Verification items for the finished model (mm, model axes). Face numbers are marked on the shaded views. A direction names the side the tool comes from. Round coordinates to 2 decimals unless told otherwise and drop trailing zeros. Order: outer loops, then holes, each group sorted by start corner. A loop starts at its lowest first (then second) coordinate and runs counter-clockwise, first axis right, second up. Notation, with made-up numbers: (30, 82.25) -> (65, 82.25) arc R6 ccw to (65, 90.25) -> close; hole circle Ø2 at (-39, 45). An arc over 180 degrees is marked (long way). Return JSON: item names as keys, results as strings. Group by question number.
Item 1: Scan lines: probe 1 along X at (y, z) = (0.5, 17); probe 2 along Y at (x, z) = (-65.6, 13.25); probe 3 along Y at (x, z) = (-19.55, 5.5). Record each from-to range of solid material in increasing order. Write a range as from..to.
Item 2: Draft check along X on the marked faces 1, 2, 3 and 4. Enter one of: pulls with the +X half, pulls with the -X half, needs draft (parallel to the pull), parting line crosses it, or undercut.
Item 3: Sectioned sample at D-D on x = 28. Record the cut outline in (y, z), plus the area to 3 significant figures.
Item 4: Depth check by flat-ended pin: pin 1 Ø5.5 at (x, y) = (-19.55, -15.5) entering from +Z; pin 2 Ø17.5 at (x, y) = (0.5, 1.5) entering from -Z; pin 3 Ø5 at (x, y) = (-65.6, -11.75) entering from -Z; pin 4 Ø2.5 at (x, y) = (-65.6, 11.75) entering from -Z. Enter the tip coordinate at first touch or a pass-through.
Item 5: Access from +Z, -Z, +X, -X, +Y, -Y to the whole of each face (thin tool, end or side, straight path). Record for the marked faces 5, 6 and 7.
Item 6: Sectioned sample at B-B on x = -65.6. Record the cut outline in (y, z).
Item 7: Sectioned sample at A-A on z = 9.4. Record the cut outline in (x, y), plus the area to 3 significant figures.
Item 8: Sectioned sample at C-C on y = 0. Give the number of separate pieces and of enclosed holes in the cut face, plus the area to 3 significant figures.
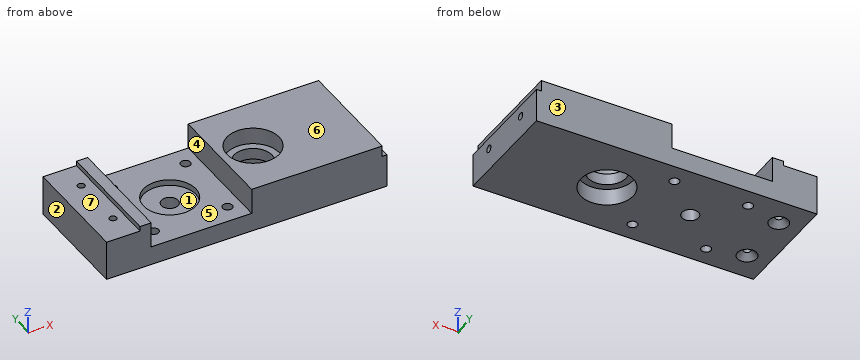
```python
from build123d import *

# Parameters (mm, degrees)
SKETCH_W        = 116
SKETCH_H        = 47
PAD_DEPTH       = 18.8
SKETCH001_R     = 4
POCKET_DEPTH    = 18.8
SKETCH029_W     = 47
SKETCH029_H     = 14.1
PAD015_DEPTH    = 2
SKETCH031_R     = 2.030946
POCKET012_DEPTH = 18.8
SKETCH032_W     = 42.3
SKETCH032_H     = 47
POCKET013_DEPTH = 10.8
SKETCH033_R     = 11
POCKET014_DEPTH = 2.5
SKETCH034_R     = 3.5
POCKET015_DEPTH = 18.801
SKETCH035_W     = 14.1
SKETCH035_H     = 47
POCKET016_DEPTH = 2
SKETCH038_R     = 11
POCKET017_DEPTH = 7
SKETCH039_R     = 11
POCKET018_DEPTH = 7
SKETCH040_R     = 8
POCKET019_DEPTH = 11.801
SKETCH072_R     = 1.5
POCKET027_DEPTH = 18.801
CHAMFER002_SIZE = 2.5
SKETCH075_R     = 1.5
POCKET030_DEPTH = 19.2


with BuildPart() as part:
    # Sketch → Pad (new body)
    with BuildSketch(Plane.XY):
        with Locations((-17, 0)):
            Rectangle(SKETCH_W, SKETCH_H)
    extrude(amount=PAD_DEPTH)

    # Sketch001 (on Face6 of Pad) → Pocket (cut)
    with BuildSketch(Plane.XY.offset(18.8)):
        Circle(SKETCH001_R)
    extrude(amount=-POCKET_DEPTH, mode=Mode.SUBTRACT)

    # Sketch029 (on Face2 of Pad) → Pad015 (join)
    with BuildSketch(Plane.YZ.offset(41)):
        with Locations((0, 7.05)):
            Rectangle(SKETCH029_W, SKETCH029_H)
    extrude(amount=PAD015_DEPTH)

    # Sketch031 (on Face4 of Pad015) → Pocket012 (cut)
    with BuildSketch(Plane(origin=(0, 0, 0), x_dir=(1, 0, 0), z_dir=(0, 0, -1))):
        with Locations((-50.55, 15.5)):
            Circle(SKETCH031_R)
        with Locations((-19.55, 15.5)):
            Circle(SKETCH031_R)
        with Locations((-50.55, -15.5)):
            Circle(SKETCH031_R)
        with Locations((-19.55, -15.5)):
            Circle(SKETCH031_R)
    extrude(amount=-POCKET012_DEPTH, mode=Mode.SUBTRACT)

    # Sketch032 (on Face5 of Pocket012) → Pocket013 (cut)
    with BuildSketch(Plane.XY.offset(18.8)):
        with Locations((-35.05, 0)):
            Rectangle(SKETCH032_W, SKETCH032_H)
    extrude(amount=-POCKET013_DEPTH, mode=Mode.SUBTRACT)

    # Sketch033 (on Face7 of Pocket013) → Pocket014 (cut)
    with BuildSketch(Plane.XY.offset(8)):
        with Locations((-35.05, 0)):
            Circle(SKETCH033_R)
    extrude(amount=-POCKET014_DEPTH, mode=Mode.SUBTRACT)

    # Sketch034 (on Face4 of Pocket014) → Pocket015 (cut, through all)
    with BuildSketch(Plane(origin=(0, 0, 0), x_dir=(1, 0, 0), z_dir=(0, 0, -1))):
        with Locations((-35.05, 0)):
            Circle(SKETCH034_R)
    extrude(amount=-POCKET015_DEPTH, mode=Mode.SUBTRACT)

    # Sketch035 (on Face5 of Pocket015) → Pocket016 (cut)
    with BuildSketch(Plane.XY.offset(18.8)):
        with Locations((-67.95, 0)):
            Rectangle(SKETCH035_W, SKETCH035_H)
    extrude(amount=-POCKET016_DEPTH, mode=Mode.SUBTRACT)

    # Sketch038 (on Face15 of Pocket016) → Pocket017 (cut)
    with BuildSketch(Plane.XY.offset(18.8)):
        Circle(SKETCH038_R)
    extrude(amount=-POCKET017_DEPTH, mode=Mode.SUBTRACT)

    # Sketch039 (on Face2 of Pocket017) → Pocket018 (cut)
    with BuildSketch(Plane(origin=(0, 0, 0), x_dir=(1, 0, 0), z_dir=(0, 0, -1))):
        Circle(SKETCH039_R)
    extrude(amount=-POCKET018_DEPTH, mode=Mode.SUBTRACT)

    # Sketch040 (on Face29 of Pocket018) → Pocket019 (cut, through all)
    with BuildSketch(Plane.XY.offset(11.8)):
        Circle(SKETCH040_R)
    extrude(amount=-POCKET019_DEPTH, mode=Mode.SUBTRACT)

    # Sketch072 (on Face2 of Pocket019) → Pocket027 (cut, through all)
    with BuildSketch(Plane(origin=(0, 0, 0), x_dir=(1, 0, 0), z_dir=(0, 0, -1))):
        with Locations((-65.6, 11.75)):
            Circle(SKETCH072_R)
        with Locations((-65.6, -11.75)):
            Circle(SKETCH072_R)
    extrude(amount=-POCKET027_DEPTH, mode=Mode.SUBTRACT)

    # Chamfer002
    chamfer002_edges = [part.edges().sort_by_distance(p)[0] for p in [
        (-67.1, -11.75, 0),
        (-67.1, 11.75, 0),
    ]]
    chamfer(chamfer002_edges, length=CHAMFER002_SIZE)

    # Sketch075 (on Face24 of Chamfer002) → Pocket030 (cut)
    with BuildSketch(Plane.YZ.offset(43)):
        with Locations((-11.75, 9.4)):
            Circle(SKETCH075_R)
        with Locations((11.75, 9.4)):
            Circle(SKETCH075_R)
    extrude(amount=-POCKET030_DEPTH, mode=Mode.SUBTRACT)


solid = part.part
```
Recorded:
{
 "1": {"probe 1": "-60.9..-56.2, -13.9..-10.99, 10.99..41", "probe 2": "-23.5..-13.25, -10.25..10.25, 13.25..23.5", "probe 3": "-23.5..-17.53, -13.47..13.47, 17.53..23.5"},
 "2": {"face 1": "undercut", "face 2": "pulls with the -X half", "face 3": "needs draft", "face 4": "undercut"},
 "3": {"outline": "(-23.5, 0) -> (23.5, 0) -> (23.5, 18.8) -> (-23.5, 18.8) -> close; hole circle Ø3 at (-11.75, 9.4); hole circle Ø3 at (11.75, 9.4)", "area": "869 mm²"},
 "4": {"pin 1": "z = 8", "pin 2": "z = 7", "pin 3": "z = 1.5", "pin 4": "through"},
 "5": {"face 5": "+Z, +Y, -Y", "face 6": "+Z, +X, -X, +Y, -Y", "face 7": "+Z, -X, +Y, -Y"},
 "6": {"outline": "(-23.5, 0) -> (-15.75, 0) -> (-13.25, 2.5) -> (-13.25, 16.8) -> (-23.5, 16.8) -> close; (-10.25, 2.5) -> (-7.75, 0) -> (7.75, 0) -> (10.25, 2.5) -> (10.25, 16.8) -> (-10.25, 16.8) -> close; (13.25, 2.5) -> (15.75, 0) -> (23.5, 0) -> (23.5, 16.8) -> (13.25, 16.8) -> close"},
 "7": {"outline": "(-75, -23.5) -> (-56.2, -23.5) -> (-56.2, 23.5) -> (-75, 23.5) -> close; (-13.9, -23.5) -> (43, -23.5) -> (43, -13.25) -> (23.8, -13.25) -> (23.8, -10.25) -> (43, -10.25) -> (43, 10.25) -> (23.8, 10.25) -> (23.8, 13.25) -> (43, 13.25) -> (43, 23.5) -> (-13.9, 23.5) -> close; hole circle Ø3 at (-65.6, -11.75); hole circle Ø3 at (-65.6, 11.75); hole circle Ø16 at (0, 0)", "area": "3,230 mm²"},
 "8": {"separate pieces": "3", "enclosed holes": "0", "area": "1,250 mm²"}
}
